```python
from build123d import *

# Parameters (mm, degrees)
BOSS_EXTRUDE1_DEPTH                             = 14.3
SKETCH2_R                                       = 1.5
CUT_EXTRUDE1_DEPTH                              = 1.3
CSK_FOR_M3_OVAL_HEAD_MACHINE_SCREW1_D           = 3.4
CSK_FOR_M3_OVAL_HEAD_MACHINE_SCREW1_CSINK_D     = 6.3
CSK_FOR_M3_OVAL_HEAD_MACHINE_SCREW1_CSINK_ANGLE = 90
BOSS_EXTRUDE2_START                             = -12.5
SKETCH8_R                                       = 6.5
BOSS_EXTRUDE2_DEPTH                             = 12.5
SKETCH14_W                                      = 40
SKETCH14_H                                      = 74
BOSS_EXTRUDE4_DEPTH                             = 25
CUT_EXTRUDE3_DEPTH                              = 4
M5_CLEARANCE_HOLE1_D                            = 5.5
FILLET1_R                                       = 4
FILLET1_OF_MIRROR3_R                            = 4
FILLET2_R                                       = 7
FILLET4_R                                       = 3
FILLET5_R                                       = 3
FILLET6_R                                       = 3
FILLET7_R                                       = 1
FILLET8_R                                       = 1
FILLET9_R                                       = 1
FILLET10_R                                      = 1
FILLET11_R                                      = 1
SKETCH21_W                                      = 13
SKETCH21_H                                      = 3.5
BOSS_EXTRUDE5_DEPTH                             = 33
CUT_EXTRUDE4_DEPTH                              = 17
CSK_FOR_M3_FLAT_HEAD_MACHINE_SCREW1_D           = 3.4
CSK_FOR_M3_FLAT_HEAD_MACHINE_SCREW1_CSINK_D     = 6.3
CSK_FOR_M3_FLAT_HEAD_MACHINE_SCREW1_CSINK_ANGLE = 90
CUT_EXTRUDE5_DEPTH                              = 434.079434689


with BuildPart() as part:
    # Sketch1 → Boss-Extrude1 (new body)
    with BuildSketch(Plane(origin=(0, 0, 0), x_dir=(1, 0, 0), z_dir=(0, 1, 0))):
        Polygon((27.724299065, -2.579662371), (27.724299065, 43.920337629), (-26.775700935, 43.920337629), (-26.775700935, 230.920337629), (27.724299065, 230.920337629), (27.724299065, 277.420337629), (-26.775700935, 277.420337629), (-26.775700935, 289.920337629), (318.224299065, 289.920337629), (318.224299065, -15.079662371), (-26.775700935, -15.079662371), (-26.775700935, -2.579662371), align=None)
    extrude(amount=BOSS_EXTRUDE1_DEPTH)

    # Sketch2 → Cut-Extrude1 (cut)
    # profile 1 of 2: a face of its own
    with BuildSketch(Plane(origin=(0, 14.3, 0), x_dir=(1, 0, 0), z_dir=(0, 1, 0))):
        Polygon((5.694299065, 191.745337629), (-9.875700935, 191.745337629), (-9.875700935, 195.230337629), (-17.275700935, 195.230337629), (-17.275700935, 171.230337629), (-9.875700935, 171.230337629), (-9.875700935, 174.715337629), (5.694299065, 174.715337629), (5.694299065, 173.570337629), (13.094299065, 173.570337629), (13.094299065, 192.890337629), (5.694299065, 192.890337629), align=None)
        with Locations(Location((-13.275700935, 191.420337629, 0), (0, 0, 270))):
            Circle(SKETCH2_R, mode=Mode.SUBTRACT)
        with Locations(Location((-13.275700935, 175.040337629, 0), (0, 0, 270))):
            Circle(SKETCH2_R, mode=Mode.SUBTRACT)
        with Locations(Location((9.094299065, 189.050337629, 0), (0, 0, 270))):
            Circle(SKETCH2_R, mode=Mode.SUBTRACT)
        with Locations(Location((9.094299065, 177.410337629, 0), (0, 0, 270))):
            Circle(SKETCH2_R, mode=Mode.SUBTRACT)
    # profile 2 of 2: a face of its own
    with BuildSketch(Plane(origin=(0, 14.3, 0), x_dir=(1, 0, 0), z_dir=(0, 1, 0))):
        Polygon((5.694299065, 100.125337629), (-9.875700935, 100.125337629), (-9.875700935, 103.610337629), (-17.275700935, 103.610337629), (-17.275700935, 79.610337629), (-9.875700935, 79.610337629), (-9.875700935, 83.095337629), (5.694299065, 83.095337629), (5.694299065, 81.950337629), (13.094299065, 81.950337629), (13.094299065, 101.270337629), (5.694299065, 101.270337629), align=None)
        with Locations(Location((-13.275700935, 99.800337629, 0), (0, 0, 270))):
            Circle(SKETCH2_R, mode=Mode.SUBTRACT)
        with Locations(Location((-13.275700935, 83.420337629, 0), (0, 0, 270))):
            Circle(SKETCH2_R, mode=Mode.SUBTRACT)
        with Locations(Location((9.094299065, 97.430337629, 0), (0, 0, 270))):
            Circle(SKETCH2_R, mode=Mode.SUBTRACT)
        with Locations(Location((9.094299065, 85.790337629, 0), (0, 0, 270))):
            Circle(SKETCH2_R, mode=Mode.SUBTRACT)
    extrude(amount=-CUT_EXTRUDE1_DEPTH, mode=Mode.SUBTRACT)

    # CSK for M3 Oval Head Machine Screw1 (through all)
    with Locations(Plane(origin=(0, 0, 0), x_dir=(-1, 0, 0), z_dir=(0, -1, 0))):
        with Locations((13.275700935, 191.420337629), (13.275700935, 175.040337629), (-9.094299065, 177.410337629), (-9.094299065, 189.050337629), (13.275700935, 83.420337629), (13.275700935, 99.800337629), (-9.094299065, 97.430337629), (-9.094299065, 85.790337629)):
            CounterSinkHole(CSK_FOR_M3_OVAL_HEAD_MACHINE_SCREW1_D / 2, CSK_FOR_M3_OVAL_HEAD_MACHINE_SCREW1_CSINK_D / 2, counter_sink_angle=CSK_FOR_M3_OVAL_HEAD_MACHINE_SCREW1_CSINK_ANGLE)

    # Sketch8 → Boss-Extrude2 (add)
    with BuildSketch(Plane.XY.offset(15.079662371).offset(BOSS_EXTRUDE2_START)):
        with BuildLine():
            Line((-26.775700935, 14.3), (73.224299065, 14.3))
            Line((73.224299065, 14.3), (31.446689864, 30.368311231))
            ThreePointArc((31.446689864, 30.368311231), (7.806182122, 37.048156923), (-16.656506763, 39.3))
            Line((-16.656506763, 39.3), (-16.775700935, 39.3))
            ThreePointArc((-16.775700935, 39.3), (-23.846768746, 36.371067812), (-26.775700935, 29.3))
            Line((-26.775700935, 29.3), (-26.775700935, 14.3))
        make_face()
        with Locations((-16.775700935, 29.3)):
            Circle(SKETCH8_R, mode=Mode.SUBTRACT)
    extrude(amount=BOSS_EXTRUDE2_DEPTH)

    # Mirror1: part across plane


with BuildPart() as part_1:
    add(part.part)
    add(part.part.mirror(Plane.XY.offset(-137.420337629)))

    # Sketch14 → Boss-Extrude4 (add)
    with BuildSketch(Plane(origin=(0, 14.3, 0), x_dir=(1, 0, 0), z_dir=(0, 1, 0))):
        with Locations((298.224299065, 21.920337629)):
            Rectangle(SKETCH14_W, SKETCH14_H)
    boss_extrude4 = extrude(amount=BOSS_EXTRUDE4_DEPTH)

    # Sketch15 → Cut-Extrude3 (cut)
    with BuildSketch(Plane(origin=(318.224299065, 0, 0), x_dir=(0, 0, -1), z_dir=(1, 0, 0))):
        Polygon((1.920337629, 24.103847577), (6.420337629, 26.701923789), (6.420337629, 31.898076211), (1.920337629, 34.496152423), (-2.579662371, 31.898076211), (-2.579662371, 26.701923789), align=None)
        Polygon((41.920337629, 24.103847577), (46.420337629, 26.701923789), (46.420337629, 31.898076211), (41.920337629, 34.496152423), (37.420337629, 31.898076211), (37.420337629, 26.701923789), align=None)
    cut_extrude3 = extrude(amount=-CUT_EXTRUDE3_DEPTH, mode=Mode.SUBTRACT)

    # M5 Clearance Hole1 (through all)
    with Locations(Plane(origin=(314.224299065, 0, 0), x_dir=(0, 0, -1), z_dir=(1, 0, 0))):
        with Locations((1.920337629, 29.3), (41.920337629, 29.3)):
            m5_clearance_hole1 = Hole(M5_CLEARANCE_HOLE1_D / 2)

    # Fillet1
    fillet1_edges = [part_1.edges().sort_by_distance(p)[0] for p in [
        (278.224299065, 39.3, -21.920337629),
    ]]
    fillet(fillet1_edges, radius=FILLET1_R)

    # Mirror3: Boss-Extrude4, Cut-Extrude3, M5 Clearance Hole1 across plane
    add(boss_extrude4.mirror(Plane.XY.offset(-137.420337629)))
    add(cut_extrude3.mirror(Plane.XY.offset(-137.420337629)), mode=Mode.SUBTRACT)
    add(m5_clearance_hole1.mirror(Plane.XY.offset(-137.420337629)), mode=Mode.SUBTRACT)

    # Fillet1 of Mirror3
    fillet1_of_mirror3_edges = [part_1.edges().sort_by_distance(p)[0] for p in [
        (278.224299065, 39.3, -252.920337629),
    ]]
    fillet(fillet1_of_mirror3_edges, radius=FILLET1_OF_MIRROR3_R)

    # Fillet2
    fillet2_edges = [part_1.edges().sort_by_distance(p)[0] for p in [
        (318.224299065, 0, -137.420337629),
    ]]
    fillet(fillet2_edges, radius=FILLET2_R)

    # Fillet4
    fillet4_edges = [part_1.edges().sort_by_distance(p)[0] for p in [
        (-26.775700935, 0, -137.420337629),
    ]]
    fillet(fillet4_edges, radius=FILLET4_R)

    # Fillet5
    fillet5_edges = [part_1.edges().sort_by_distance(p)[0] for p in [
        (-26.775700935, 0, 8.829662371),
    ]]
    fillet(fillet5_edges, radius=FILLET5_R)

    # Fillet6
    fillet6_edges = [part_1.edges().sort_by_distance(p)[0] for p in [
        (-26.775700935, 0, -283.670337629),
    ]]
    fillet(fillet6_edges, radius=FILLET6_R)

    # Fillet7
    fillet7_edges = [part_1.edges().sort_by_distance(p)[0] for p in [
        (52.335494465, 22.334155616, 15.079662371),
        (7.806182122, 37.048156923, 15.079662371),
        (-16.716103849, 39.3, 15.079662371),
        (-23.846768746, 36.371067812, 15.079662371),
        (318.224299065, 23.15, 15.079662371),
        (-26.775700935, 16.15, 15.079662371),
        (316.174046534, 2.050252532, 15.079662371),
        (143.724299065, 0, 15.079662371),
        (-25.897021278, 0.878679656, 15.079662371),
    ]]
    fillet(fillet7_edges, radius=FILLET7_R)

    # Fillet8
    fillet8_edges = [part_1.edges().sort_by_distance(p)[0] for p in [
        (-26.775700935, 16.15, -289.920337629),
        (318.224299065, 23.15, -289.920337629),
        (-23.846768746, 36.371067812, -289.920337629),
        (-16.716103849, 39.3, -289.920337629),
        (7.806182122, 37.048156923, -289.920337629),
        (52.335494465, 22.334155616, -289.920337629),
        (143.724299065, 0, -289.920337629),
        (316.174046534, 2.050252532, -289.920337629),
        (-25.897021278, 0.878679656, -289.920337629),
    ]]
    fillet(fillet8_edges, radius=FILLET8_R)

    # Fillet9
    fillet9_edges = [part_1.edges().sort_by_distance(p)[0] for p in [
        (27.724299065, 0, -20.670337629),
        (1.974299065, 0, 2.579662371),
        (-26.775700935, 8.65, -43.920337629),
        (-23.846768746, 36.371067812, 2.579662371),
        (-16.716103849, 39.3, 2.579662371),
        (7.806182122, 37.048156923, 2.579662371),
        (52.335494465, 22.334155616, 2.579662371),
        (-26.775700935, 16.15, 2.579662371),
        (1.974299065, 0, -43.920337629),
        (-25.897021278, 0.878679656, -43.920337629),
        (-25.897021278, 0.878679656, 2.579662371),
    ]]
    fillet(fillet9_edges, radius=FILLET9_R)

    # Fillet10
    fillet10_edges = [part_1.edges().sort_by_distance(p)[0] for p in [
        (1.974299065, 0, -230.920337629),
        (27.724299065, 0, -254.170337629),
        (-26.775700935, 8.65, -230.920337629),
        (-26.775700935, 16.15, -277.420337629),
        (52.335494465, 22.334155616, -277.420337629),
        (7.806182122, 37.048156923, -277.420337629),
        (-16.716103849, 39.3, -277.420337629),
        (-23.846768746, 36.371067812, -277.420337629),
        (-25.897021278, 0.878679656, -230.920337629),
        (1.974299065, 0, -277.420337629),
        (-25.897021278, 0.878679656, -277.420337629),
    ]]
    fillet(fillet10_edges, radius=FILLET10_R)

    # Fillet11
    fillet11_edges = [part_1.edges().sort_by_distance(p)[0] for p in [
        (0.974299065, 14.3, -230.920337629),
        (0.974299065, 14.3, -43.920337629),
        (-26.482807716, 14.3, -44.213230848),
        (-26.775700935, 14.3, -137.420337629),
        (-26.482807716, 14.3, -230.62744441),
    ]]
    fillet(fillet11_edges, radius=FILLET11_R)

    # Sketch21 → Boss-Extrude5 (add)
    with BuildSketch(Plane(origin=(0, 14.3, 0), x_dir=(1, 0, 0), z_dir=(0, 1, 0))):
        with Locations((215.599299065, 13.170337629)):
            Rectangle(SKETCH21_W, SKETCH21_H)
        with Locations((215.599299065, 26.670337629)):
            Rectangle(SKETCH21_W, SKETCH21_H)
    boss_extrude5 = extrude(amount=BOSS_EXTRUDE5_DEPTH)

    # Sketch22 → Cut-Extrude4 (cut)
    with BuildSketch(Plane.XY.offset(-11.420337629)):
        with BuildLine():
            Line((209.099299065, 41.3), (209.099299065, 47.3))
            Line((209.099299065, 47.3), (215.599299065, 49.081376358))
            Line((215.599299065, 49.081376358), (222.099299065, 47.3))
            Line((222.099299065, 47.3), (222.099299065, 41.3))
            ThreePointArc((222.099299065, 41.3), (215.599299065, 47.3), (209.099299065, 41.3))
        make_face()
    cut_extrude4 = extrude(amount=-CUT_EXTRUDE4_DEPTH, mode=Mode.SUBTRACT)

    # CSK for M3 Flat Head Machine Screw1 (through all)
    with Locations(Plane.XY.offset(-11.420337629)):
        with Locations((215.594856714, 41.29339707), (185.090080481, 50.471650395), (10.649939144, 122.619059121)):
            csk_for_m3_flat_head_machine_screw1 = CounterSinkHole(CSK_FOR_M3_FLAT_HEAD_MACHINE_SCREW1_D / 2, CSK_FOR_M3_FLAT_HEAD_MACHINE_SCREW1_CSINK_D / 2, counter_sink_angle=CSK_FOR_M3_FLAT_HEAD_MACHINE_SCREW1_CSINK_ANGLE)

    # Mirror4: Boss-Extrude5, Cut-Extrude4, CSK for M3 Flat Head Machine Screw1 across plane
    add(boss_extrude5.mirror(Plane.XY.offset(-137.420337629)))
    add(cut_extrude4.mirror(Plane.XY.offset(-137.420337629)), mode=Mode.SUBTRACT)
    add(csk_for_m3_flat_head_machine_screw1.mirror(Plane.XY.offset(-137.420337629)), mode=Mode.SUBTRACT)

    # only_engine_part → Cut-Extrude5 (cut, through all)
    with BuildSketch(Plane.XZ):
        Polygon((-26.775700935, -289.920337629), (318.224299065, -289.920337629), (318.224299065, 15.079662371), (63.094299065, 15.079662371), (63.094299065, -132.610337629), (-26.775700935, -132.610337629), align=None)
    extrude(amount=-CUT_EXTRUDE5_DEPTH, mode=Mode.SUBTRACT)


solid = part_1.part
```
Verification items for the finished model (mm, model axes). A direction names the side the tool comes from. Give positions to 0.01 mm unless a question says otherwise; leave off trailing zeros. Order: outer loops, then holes, each group sorted by start corner. A loop starts at its lowest first (then second) coordinate and runs counter-clockwise, first axis right, second up. Notation, with made-up numbers: (35, -27.75) -> (65, -27.75) arc R31 ccw to (65, 7.25) -> close; hole circle Ø1 at (47.5, 74.5). An arc over 180 degrees is marked (long way). One line per item, written item: value.
(1) Sectioned sample at B-B on z = -9. Record the cut outline in (x, y), then the cut area to 3 significant figures.
Final values:
outline: (27.72, 1) arc R1 ccw to (28.72, 0) -> (63.09, 0) -> (63.09, 14.3) -> (27.72, 14.3) -> close
area: 506 mm^2
(2) Tool access check on faces 1 (the face through (63.094, 7, -58)), 2 (the face through (1, 7, -43.92)). Record the directions out of +Z, -Z, +X, -X, +Y, -Y that give a thin tool (end or side, any length) a straight path to the whole face; none if there is none.
Final values:
face 1: +Z, -Z, +X, +Y, -Y
face 2: -X, +Y, -Y
(3) Draft check along Y on faces 3 (the face through (20, 0, -60)), 4 (the face through (7.396, 7.306, -97.505)), 5 (the face through (-10.77, 26.81, 8.74)), 6 (the face through (47.124, 24.033, 2.88)). Enter one of: pulls with the +Y half, pulls with the -Y half, needs draft (parallel to the pull), parting line crosses it, or undercut.
Final values:
face 3: pulls with the -Y half
face 4: needs draft
face 5: undercut
face 6: pulls with the +Y half
(4) Sectioned sample at D-D on z = -116. Record the cut outline in (x, y), then the cut area to 3 significant figures.
Final values:
outline: (-26.78, 3) arc R3 ccw to (-23.78, 0) -> (63.09, 0) -> (63.09, 14.3) -> (-25.78, 14.3) arc R1 ccw to (-26.78, 13.3) -> close
area: 1,280 mm^2
(5) Sectioned sample at C-C on x = -19. Count the separate pieces of the cut face and the enclosed holes in it, then the cut area to 3 significant figures.
Final values:
separate pieces: 3
enclosed holes: 0
area: 1,600 mm^2
(6) Scan lines: line 1 along Y through (x, z) = (9, -104.5); line 2 along X through (y, z) = (3, -5); line 3 along Z through (x, y) = (0, 31.5). Record each from-to range of solid material in increasing order. Write a range as [from, to].
Final values:
line 1: [0, 14.3]
line 2: [27.72, 63.09]
line 3: [2.58, 15.08]
(7) Gauge pin test, flat ends, axial feed: pin 1 (12 mm diameter, centred on x = 29.5, y = 33.5, fed in from -Z); pin 2 (0.7 mm diameter, centred on y = 14, z = -101, fed in from -X). Record the tip position at first contact, or that the pin passes through.
Final values:
pin 1: z = 2.58
pin 2: x = -26.71
(8) Sectioned sample at A-A on y = 11. Record the cut outline in (x, z).
Final values:
outline: (-26.78, -132.61) -> (63.09, -132.61) -> (63.09, 15.08) -> (-25.78, 15.08) arc R1 ccw to (-26.78, 14.08) -> (-26.78, 3.58) arc R1 ccw to (-25.78, 2.58) -> (27.72, 2.58) -> (27.72, -43.92) -> (-25.78, -43.92) arc R1 ccw to (-26.78, -44.92) -> close; hole circle Ø3.4 at (-13.28, -99.8); hole circle Ø3.4 at (-13.28, -83.42); hole circle Ø3.4 at (9.09, -97.43); hole circle Ø3.4 at (9.09, -85.79)
